Source: three-view drawing plus pictorial views. Frame: mm from the lowest corner of the part. A direction names the side the tool comes from. Round coordinates to 2 decimals unless told otherwise and drop trailing zeros. Loops run counter-clockwise (first coordinate to the right, second up) from the corner with the lowest first, then second, coordinate; pieces in that order, holes last. Notation, with made-up numbers: (0.25, 13.5) -> (42.25, 13.5) arc R22 ccw to (42.25, 29.5) -> close; hole circle Ø9 at (27, 38). An arc over 180 degrees is marked (long way). Return JSON: item names as keys, results as strings. Group by question number.
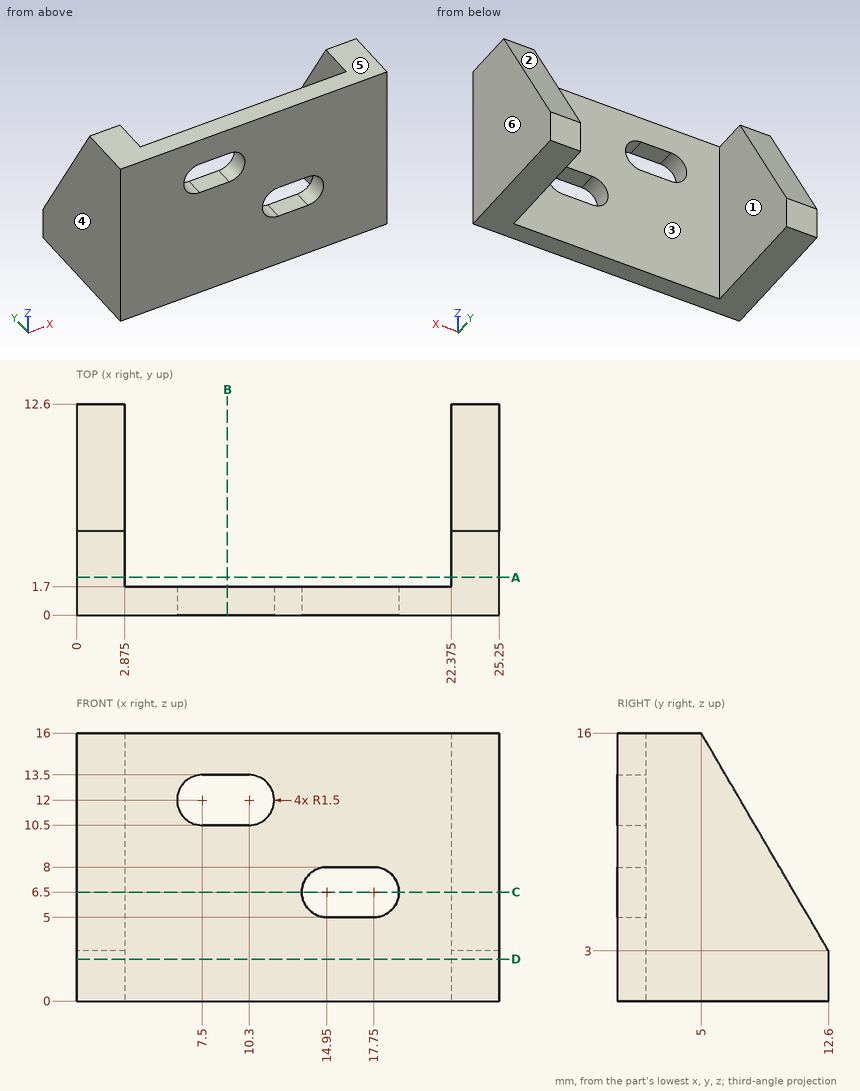
(1) Ray query, line 1 (X direction, y = 5.75, z = 1) (3 decimals); line 2 (Z direction, x = 10, y = 1.5); line 3 (Y direction, x = 21.5, z = 8). Return the intervals inside material, ascending.
(2) Cut plane B-B (x = 9). Return loops of the section in (y, z).
(3) Cut plane A-A (y = 2.25). Return loops of the section in (x, z) (3 decimals), and give its area (3 significant figures).
(4) Cut plane D-D (z = 2.5). Return loops of the section in (x, y) (3 decimals).
(5) Pin query (flat end, axial travel): pin 1 (4 mm diameter, centred on x = 8.5, z = 12.5, fed in from +Y); pin 2 (3 mm diameter, centred on x = 20.5, y = 8, fed in from -Z). Return the tip coordinate at first contact, or that it passes through.
(6) Cut plane C-C (z = 6.5). Return loops of the section in (x, y) (3 decimals), and give its area (3 significant figures).
(7) Mould query, pull axis X, two halves, no side actions, for the marked faces 3, 4, 5 and 6. Classes: released by +X, released by -X, zero draft, split by the parting line, or undercut.
(8) Set-up query: the marked faces 1 and 2. Return all of +Z, -Z, +X, -X, +Y, -Y with unobstructed straight access to the full face (end or side cutting, diameter ignored); none if empty.
Answers follow:
{
 "1": {"line 1": "0 to 2.875, 22.375 to 25.25", "line 2": "0 to 10.5, 13.5 to 16", "line 3": "0 to 1.7"},
 "2": {"outline": "(0, 0) -> (1.7, 0) -> (1.7, 10.5) -> (0, 10.5) -> close; (0, 13.5) -> (1.7, 13.5) -> (1.7, 16) -> (0, 16) -> close"},
 "3": {"outline": "(0, 0) -> (2.875, 0) -> (2.875, 16) -> (0, 16) -> close; (22.375, 0) -> (25.25, 0) -> (25.25, 16) -> (22.375, 16) -> close", "area": "92.0 mm^2"},
 "4": {"outline": "(0, 0) -> (25.25, 0) -> (25.25, 12.6) -> (22.375, 12.6) -> (22.375, 1.7) -> (2.875, 1.7) -> (2.875, 12.6) -> (0, 12.6) -> close"},
 "5": {"pin 1": "y = 1.7", "pin 2": "through"},
 "6": {"outline": "(0, 0) -> (13.45, 0) -> (13.45, 1.7) -> (2.875, 1.7) -> (2.875, 10.554) -> (0, 10.554) -> close; (19.25, 0) -> (25.25, 0) -> (25.25, 10.554) -> (22.375, 10.554) -> (22.375, 1.7) -> (19.25, 1.7) -> close", "area": "84.0 mm^2"},
 "7": {"face 3": "undercut", "face 4": "released by -X", "face 5": "zero draft", "face 6": "released by +X"},
 "8": {"face 1": "+Z, -Z, +Y", "face 2": "+Z, +X, -X, +Y"}
}
